Autodesk Fusion 360 part; units mm, degrees
sketch "Sketch1" plane through (0, 0, 0) normal (0, 1, 0) x (1, 0, 0) in component "softJaws"
  line L0 (0, 0) -> (127, 0)
  line L1 (127, 0) -> (127, -38.1)
  line L2 (127, -38.1) -> (0, -38.1)
  line L3 (0, -38.1) -> (0, 0)
  circle A0 centre (23.8125, -21.59) radius 5.715
  line L4 (23.8125, -21.59) -> (103.1875, -21.59) construction
  circle A1 centre (103.1875, -21.59) radius 5.715
  line L5 (63.5, -38.1) -> (63.5, 0) construction
  point P0 (63.5, -21.59)
  dimension "d1" = 127
  dimension "d2" = 38.1
  dimension "d3" = 11.43
  dimension "d4" = 21.59
  dimension "d6" = 79.375
  dimension "d7" = 11.43
extrude "Extrude1" add sketch "Sketch1" along normal blind 19.05 in component "softJaws"
sketch "Sketch2" plane through (0, 0, 0) normal (0, -1, 0) x (1, 0, 0) in component "softJaws"
  circle A0 centre (103.1875, 21.59) radius 5.715
  circle A1 centre (23.8125, 21.59) radius 5.715
  line L0 (127, 38.1) -> (0, 38.1)
  line L1 (0, 38.1) -> (0, 0)
  line L2 (0, 0) -> (127, 0)
  line L3 (127, 0) -> (127, 38.1)
  circle A2 centre (23.8125, 21.59) radius 8.89
  circle A3 centre (103.1875, 21.59) radius 8.89
  dimension "d10" = 17.78
  dimension "d11" = 17.78
extrude "Extrude2" cut sketch "Sketch2" against normal blind 12.7 contours A2 | A3 in component "softJaws"
component "softJaws" placed x (1, 0, 0) y (0, 1, 0) z (0, 0, 1) at (0, 0, 0)
equation "d4 = d2 / 2 + 0.1 in"
Design review of the part built by this model. Coordinates are the model's own, in mm. A direction names the side the tool comes from. Coordinates: 2 decimals unless noted, no trailing zeros. Loops run counter-clockwise (first coordinate to the right, second up) from the corner with the lowest first, then second, coordinate; pieces in that order, holes last. Notation, with made-up numbers: (-33.75, 14.25) - (-17.75, 14.25) arc R20 ccw to (-17.75, 38.25) - close; hole circle Ø5 at (51.25, 59). An arc over 180 degrees is marked (long way). Use CSV: the item, a comma, the result in double quotes. Start each with the question number.
1. Mouldability with a two-part tool opening along Z and no side actions: class faces 1 (the flat face through (63, 9, 0)), 2 (the flat face through (63, 19.05, 19)), 3 (the cylindrical face through (19.6, 15.83, 25.45)) as released by +Z, released by -Z, zero draft, split by the parting line, or undercut.
2. To check wall thickness, follow probe 1 along X at (y, z) = (5.5, 27.5); probe 2 along X at (y, z) = (16.5, 25); probe 3 along Z at (x, y) = (108, 8.75). State the ranges of each line that lie inside material, in increasing order.
3. For faces 4 (the flat face through (63, 0, 19)), 5 (the flat face through (109, 12.7, 20)), list the 3-axis set-ups (+Z, -Z, +X, -X, +Y, -Y) from which the entire face can be reached by the end or side of a thin tool; tool diameter is ignored.
4. Clearance check with flat-ended pins moving along their axes: pin 1 (14 mm diameter, centred on x = 103.19, z = 21.59, fed in from +Y); pin 2 (10.5 mm diameter, centred on x = 23.81, z = 21.59, fed in from +Y). State where each tip first meets the part, or that it passes through.
5. Add section A-A on z = 21.59. Give the boundary of the cut face in (x, y).
6. Add section B-B on y = 3. Give the boundary of the cut face in (x, z), plus the area to 3 significant figures.
Resolved:
1,face 1,"released by -Z"
1,face 2,"zero draft"
1,face 3,"undercut"
2,probe 1,"0 to 17.17, 30.45 to 96.55, 109.83 to 127"
2,probe 2,"0 to 19.23, 28.4 to 98.6, 107.77 to 127"
2,probe 3,"0 to 14.12, 29.06 to 38.1"
3,face 4,"+Z, -Z, +X, -X, -Y"
3,face 5,"-Y"
4,pin 1,"y = 19.05"
4,pin 2,"through"
5,outline,"(0, 0) - (14.92, 0) - (14.92, 12.7) - (18.1, 12.7) - (18.1, 19.05) - (0, 19.05) - close; (29.53, 12.7) - (32.7, 12.7) - (32.7, 0) - (94.3, 0) - (94.3, 12.7) - (97.47, 12.7) - (97.47, 19.05) - (29.53, 19.05) - close; (108.9, 12.7) - (112.08, 12.7) - (112.08, 0) - (127, 0) - (127, 19.05) - (108.9, 19.05) - close"
6,outline,"(0, 0) - (127, 0) - (127, 38.1) - (0, 38.1) - close; hole circle Ø17.78 at (23.81, 21.59); hole circle Ø17.78 at (103.19, 21.59)"
6,area,"4,340 mm2"
